from build123d import *

# Parameters (mm, degrees)
SKETCH_1_W          = 10
SKETCH_1_H          = 15
SKETCH_1_W_2        = 8.666666666
SKETCH_1_H_2        = 13
EXTRUDE_1_DEPTH     = 56.5
SKETCH_2_R          = 1.6
CUT_EXTRUDE_1_DEPTH = 58.866225037
SKETCH_3_R          = 1.6
CUT_EXTRUDE_2_DEPTH = 59.67069115
SKETCH_4_R          = 1.6
CUT_EXTRUDE_3_DEPTH = 58.866225037


with BuildPart() as part:
    # ｽｹｯﾁ1 → ﾎﾞｽ - 押し出し1 (new body)
    with BuildSketch(Plane.XY):
        Rectangle(SKETCH_1_W, SKETCH_1_H)
        Rectangle(SKETCH_1_W_2, SKETCH_1_H_2, mode=Mode.SUBTRACT)
    extrude_1 = extrude(amount=EXTRUDE_1_DEPTH)

    # ｽｹｯﾁ2 → ｶｯﾄ - 押し出し1 (cut, through all)
    with BuildSketch(Plane(origin=(5, 0, 0), x_dir=(0, 0, -1), z_dir=(1, 0, 0))):
        Circle(SKETCH_2_R)
    cut_extrude_1 = extrude(amount=-CUT_EXTRUDE_1_DEPTH, mode=Mode.SUBTRACT)

    # ｽｹｯﾁ3 → ｶｯﾄ - 押し出し2 (cut, through all)
    with BuildSketch(Plane(origin=(0, 7.5, 0), x_dir=(1, 0, 0), z_dir=(0, 1, 0))):
        with Locations(Location((0, -51.5, 0), (0, 0, 270))):
            Circle(SKETCH_3_R)
    cut_extrude_2 = extrude(amount=-CUT_EXTRUDE_2_DEPTH, mode=Mode.SUBTRACT)

    # ｽｹｯﾁ4 → ｶｯﾄ - 押し出し3 (cut, through all)
    with BuildSketch(Plane.ZY.offset(5)):
        with Locations((51.5, 0)):
            Circle(SKETCH_4_R)
    cut_extrude_3 = extrude(amount=-CUT_EXTRUDE_3_DEPTH, mode=Mode.SUBTRACT)

    # ﾐﾗｰ1: ﾎﾞｽ - 押し出し1, ｶｯﾄ - 押し出し1, ｶｯﾄ - 押し出し2, ｶｯﾄ - 押し出し3 across plane
    add(extrude_1.mirror(Plane(origin=(0, 0, 0), x_dir=(1, 0, 0), z_dir=(0, 0, -1))))
    add(cut_extrude_1.mirror(Plane(origin=(0, 0, 0), x_dir=(1, 0, 0), z_dir=(0, 0, -1))), mode=Mode.SUBTRACT)
    add(cut_extrude_2.mirror(Plane(origin=(0, 0, 0), x_dir=(1, 0, 0), z_dir=(0, 0, -1))), mode=Mode.SUBTRACT)
    add(cut_extrude_3.mirror(Plane(origin=(0, 0, 0), x_dir=(1, 0, 0), z_dir=(0, 0, -1))), mode=Mode.SUBTRACT)


solid = part.part
Check sheet for the modelled part. Datum: model origin and axes. Units: mm. A direction names the side the tool comes from. Coordinates: 2 decimals unless noted, no trailing zeros. Loops run counter-clockwise (first coordinate to the right, second up) from the corner with the lowest first, then second, coordinate; pieces in that order, holes last. Notation, with made-up numbers: (31, 23) -> (68, 23) arc R22 ccw to (68, 53) -> close; hole circle Ø5 at (37.25, 35). An arc over 180 degrees is marked (long way). Answer in a Markdown table with one row per item.
1. Sectioned sample at D-D, the plane x = 0. Record the boundary of the cut face in (y, z).
Check values:
| item | result |
|---|---|
| outline | (-7.5, -56.5) -> (-6.5, -56.5) -> (-6.5, -53.1) -> (-7.5, -53.1) -> close; (-7.5, -49.9) -> (-6.5, -49.9) -> (-6.5, 49.9) -> (-7.5, 49.9) -> close; (-7.5, 53.1) -> (-6.5, 53.1) -> (-6.5, 56.5) -> (-7.5, 56.5) -> close; (6.5, -56.5) -> (7.5, -56.5) -> (7.5, -53.1) -> (6.5, -53.1) -> close; (6.5, -49.9) -> (7.5, -49.9) -> (7.5, 49.9) -> (6.5, 49.9) -> close; (6.5, 53.1) -> (7.5, 53.1) -> (7.5, 56.5) -> (6.5, 56.5) -> close |
2. Sectioned sample at B-B, the plane z = 0. Record the boundary of the cut face in (x, y), then the cut area to 3 significant figures.
Check values:
| item | result |
|---|---|
| outline | (-5, -7.5) -> (5, -7.5) -> (5, -1.6) -> (4.33, -1.6) -> (4.33, -6.5) -> (-4.33, -6.5) -> (-4.33, -1.6) -> (-5, -1.6) -> close; (-5, 1.6) -> (-4.33, 1.6) -> (-4.33, 6.5) -> (4.33, 6.5) -> (4.33, 1.6) -> (5, 1.6) -> (5, 7.5) -> (-5, 7.5) -> close |
| area | 33.1 mm2 |
3. Access from +Z, -Z, +X, -X, +Y, -Y to the whole of each face (thin tool, end or side, straight path). Record for faces 5 (the face through (4.333, -2, 1)), 6 (the face through (0, 7.5, 1)).
Check values:
| item | result |
|---|---|
| face 5 | +Z, -Z |
| face 6 | +Z, -Z, +X, -X, +Y |
4. Go/stop test with a flat-tipped pin: pin 1 (2.5 mm diameter, centred on y = 0, z = 51.5, fed in from +X). Record where the tip stops, or that it passes through.
Check values:
| item | result |
|---|---|
| pin 1 | passes through |
5. Sectioned sample at A-A, the plane y = 0. Give the number of separate pieces and of enclosed holes in the cut face, then the cut area to 3 significant figures.
Check values:
| item | result |
|---|---|
| separate pieces | 8 |
| enclosed holes | 0 |
| area | 138 mm2 |
6. Release check for a two-part mould opening along Z. For faces 1 (the face through (0.481, 7.007, 53.026)), 2 (the face through (5, -2, 1)), 3 (the face through (-4.671, 0.481, -53.026)), 4 (the face through (-4.5, 0.1, -56.5)) record: released by +Z, released by -Z, zero draft, split by the parting line, or undercut.
Check values:
| item | result |
|---|---|
| face 1 | undercut |
| face 2 | zero draft |
| face 3 | undercut |
| face 4 | released by -Z |
7. Sectioned sample at C-C, the plane z = 25. Record the boundary of the cut face in (x, y), then the cut area to 3 significant figures.
Check values:
| item | result |
|---|---|
| outline | (-5, -7.5) -> (5, -7.5) -> (5, 7.5) -> (-5, 7.5) -> close; hole (-4.33, -6.5) -> (4.33, -6.5) -> (4.33, 6.5) -> (-4.33, 6.5) -> close |
| area | 37.3 mm2 |
8. Material ranges on line 1 along Y through (x, z) = (0.5, -13); line 2 along X through (y, z) = (5.25, -22.5); line 3 along X through (y, z) = (6.85, -51.5), recorded low to high. Write a range as [from, to].
Check values:
| item | result |
|---|---|
| line 1 | y = [-7.5, -6.5], [6.5, 7.5] |
| line 2 | x = [-5, -4.33], [4.33, 5] |
| line 3 | x = [-5, -1.6], [1.6, 5] |
